```python
from build123d import *

# Parameters (mm, degrees)
SKETCH1_R           = 4.7625
BOSS_EXTRUDE1_DEPTH = 5


with BuildPart() as part:
    # Sketch1 → Boss-Extrude1 (new body)
    with BuildSketch(Plane.XY):
        with BuildLine():
            Line((-11.599180508, 2.297223602), (-11.599180508, -0.562353553))
            Line((-11.599180508, -0.562353553), (-11.599180508, -3.961142474))
            Line((-11.599180508, -3.961142474), (13.644266696, -3.961142474))
            Line((13.644266696, -3.961142474), (13.644266696, -0.562353553))
            Line((13.644266696, -0.562353553), (13.644266696, 2.297223602))
            ThreePointArc((13.644266696, 2.297223602), (11.528131098, 5.464244333), (10.785043094, 9.2))
            ThreePointArc((10.785043094, 9.2), (1.022543094, 18.9625), (-8.739956906, 9.2))
            ThreePointArc((-8.739956906, 9.2), (-9.48304491, 5.464244333), (-11.599180508, 2.297223602))
        make_face()
        with Locations((1.022543094, 9.2)):
            Circle(SKETCH1_R, mode=Mode.SUBTRACT)
    extrude(amount=BOSS_EXTRUDE1_DEPTH)


solid = part.part
```
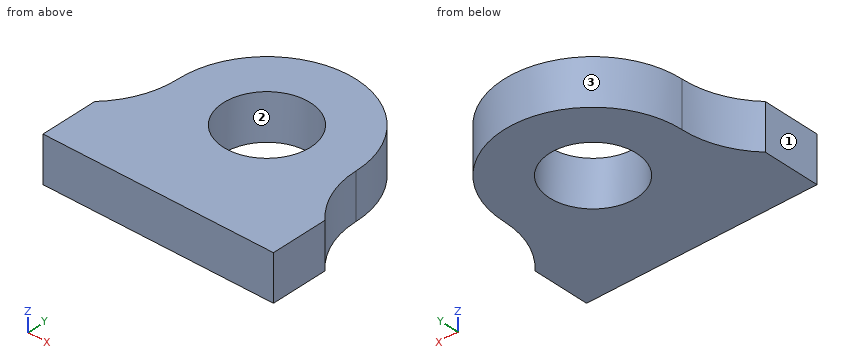
Input: part model. Units: mm. Frame: model coordinates. Face numbers are marked on the shaded views. Coordinates: 2 decimals unless noted, no trailing zeros. Loops run counter-clockwise (first coordinate to the right, second up) from the corner with the lowest first, then second, coordinate; pieces in that order, holes last. Notation, with made-up numbers: M 10.25,-28.75 L 24.25,-28.75 A25 ccw 24.25,9.25 Z; hole C 0.25,84 d3. An arc over 180 degrees is marked long. Use a Markdown table: item, result. Add a question column.
1) Draft query along Y for the marked faces 1, 2 and 3. Return one class per face: +Y half, -Y half, draft (parallel to the pull), parting line (faces both ways), or undercut.
2) Pin query (flat end, axial travel): P1, Ø1, axis at x = -6, z = 1, coming from the +Y side; P2, Ø1, axis at x = 4, z = 2.5, coming from the +Y side; P3, Ø12, axis at x = 6.5, y = 0, coming from the -Z side. Return the tip coordinate at first contact, or that it passes through.
3) Section D-D, the plane x = 7. Return the cut outline in (y, z), plus the area to 3 significant figures.
4) Line query: L1, parallel to Y at x = 3.25, z = 3.75 (1 decimal); L2, parallel to Y at x = 5.25, z = 4.65; L3, parallel to X at y = 5, z = 4.4. Output: solid intervals per line, ascending. Write a range as from..to.
5) Section C-C, the plane x = 2.25. Return the cut outline in (y, z), plus the area to 3 significant figures.
6) Section B-B, the plane y = 6. Return the cut outline in (x, z), plus the area to 3 significant figures.
Answer below:
| question | item | result |
|---|---|---|
| 1 | face 1 | draft |
| 1 | face 2 | undercut |
| 1 | face 3 | +Y half |
| 2 | P1 | y = 16.46 |
| 2 | P2 | y = 18.64 |
| 2 | P3 | z = 0 |
| 3 | outline | M -3.96,0 L 16.92,0 L 16.92,5 L -3.96,5 Z |
| 3 | area | 104 mm2 |
| 4 | L1 | -4..5, 13.4..18.7 |
| 4 | L2 | -3.96..7.01, 11.39..18 |
| 4 | L3 | -9.69..-1.22, 3.27..11.73 |
| 5 | outline | M -3.96,0 L 4.6,0 L 4.6,5 L -3.96,5 Z; M 13.8,0 L 18.89,0 L 18.89,5 L 13.8,5 Z |
| 5 | area | 68.2 mm2 |
| 6 | outline | M -9.28,0 L -2.5,0 L -2.5,5 L -9.28,5 Z; M 4.55,0 L 11.32,0 L 11.32,5 L 4.55,5 Z |
| 6 | area | 67.7 mm2 |
